For this review, take the finished solid that the model builds, in its own axes (mm). Give positions to 0.01 mm unless a question says otherwise; leave off trailing zeros. Loops run counter-clockwise (first coordinate to the right, second up) from the corner with the lowest first, then second, coordinate; pieces in that order, holes last. Notation, with made-up numbers: (81, 65.5) -> (119, 65.5) arc R19 cw to (119, 69.5) -> close; hole circle Ø10 at (-6.75, 21). An arc over 180 degrees is marked (long way). One line per question, with ' | ' between items. Start each with the question number.
(1) Consider section B-B (y = 1384). Write out the cut boundary in (x, z), and give its area (3 significant figures).
(2) Wall thickness on probe 1 along X at (y, z) = (106.5, 14.75); probe 2 along X at (y, z) = (53.5, 5.25); probe 3 along X at (y, z) = (476, 17.5): over which ranges is each line inside the solid? List them lowest first.
(3) Consider section C-C (x = -246). Write out the cut boundary in (y, z), and give its area (3 significant figures).
(4) Consider section A-A (z = 12). Give the number of separate pieces and of enclosed holes in the cut face, and give its area (3 significant figures).
(5) Insertion check: P1, Ø1.5, axis at y = 1042, z = 14, coming from the -X side; P2, Ø8, axis at y = 1371.5, z = 5, coming from the -X side; P3, Ø10, axis at x = -301, z = 5.5, coming from the +Y side. Each pin has a flat end and moves straight along its axis. Give the tip position at first contact, or say it passes through.
from build123d import *

# Parameters (mm, degrees)
F0_W     = 19.812
F0_H     = 50.8
F0_W_2   = 19.05
F0_H_2   = 38.1
F1_DEPTH = 19.812
F2_R     = 12.7
F3_DEPTH = 254


# Not quite as in the source:
# - a feature names something its author has since deleted; it is built from what else it names


with BuildPart() as f1:
    # F0 (on Top) → F1 (new body)
    with BuildSketch(Plane.XY):
        Polygon((-468.2972775146, 751.1484609425), (-468.2972775146, -61.6515390575), (-61.8972775146, -61.6515390575), (-61.8972775146, 166.9484609425), (39.7027224854, 166.9484609425), (39.7027224854, -61.6515390575), (446.1027224854, -61.6515390575), (446.1027224854, 751.1484609425), (141.3027224854, 1411.5484609425), (141.3027224854, 1614.7484609425), (-11.0972775146, 1614.7484609425), (-163.4972775146, 1614.7484609425), (-163.4972775146, 1411.5484609425), align=None)
        with Locations((-439.3412775146, 14.5484609425)):
            Rectangle(F0_W, F0_H, mode=Mode.SUBTRACT)
        with Locations((-439.3412775146, 116.1484609425)):
            Rectangle(F0_W, F0_H, mode=Mode.SUBTRACT)
        with Locations((417.1467224854, 14.5484609425)):
            Rectangle(F0_W, F0_H, mode=Mode.SUBTRACT)
        with Locations((417.1467224854, 116.1484609425)):
            Rectangle(F0_W, F0_H, mode=Mode.SUBTRACT)
        with Locations((328.6277224854, 465.3984609425)):
            Rectangle(F0_W_2, F0_H_2, mode=Mode.SUBTRACT)
    extrude(amount=F1_DEPTH)

    # F2 (on face) → F3 (cut)
    with BuildSketch(Plane.XY.offset(19.812)):
        with Locations((-11.0972775146, 1513.1484609425)):
            Circle(F2_R)
    extrude(amount=-F3_DEPTH, mode=Mode.SUBTRACT)


solid = f1.part
A:
1) outline: (-176.21, 0) -> (154.02, 0) -> (154.02, 19.81) -> (-176.21, 19.81) -> close | area: 6,540 mm^2
2) probe 1: x = -468.3 to -449.25, -429.44 to -61.9, 39.7 to 407.24, 427.05 to 446.1 | probe 2: x = -468.3 to -61.9, 39.7 to 446.1 | probe 3: x = -468.3 to 319.1, 338.15 to 446.1
3) outline: (-61.65, 0) -> (1232.79, 0) -> (1232.79, 19.81) -> (-61.65, 19.81) -> close | area: 25,600 mm^2
4) separate pieces: 1 | enclosed holes: 6 | area: 1,180,000 mm^2
5) P1: stops at x = -334.4 | P2: stops at x = -183.83 | P3: stops at y = 1124.46
